Geometry: final body of the model. Coordinates: model frame, mm. Face numbers are marked on the shaded views. A direction names the side the tool comes from. Round coordinates to 2 decimals unless told otherwise and drop trailing zeros. Loops run counter-clockwise (first coordinate to the right, second up) from the corner with the lowest first, then second, coordinate; pieces in that order, holes last. Notation, with made-up numbers: M 30,13.25 L 55,13.25 A14 cw 55,26.25 Z; hole C 8,-7.75 d1. An arc over 180 degrees is marked long. Return JSON: item names as keys, results as strings.
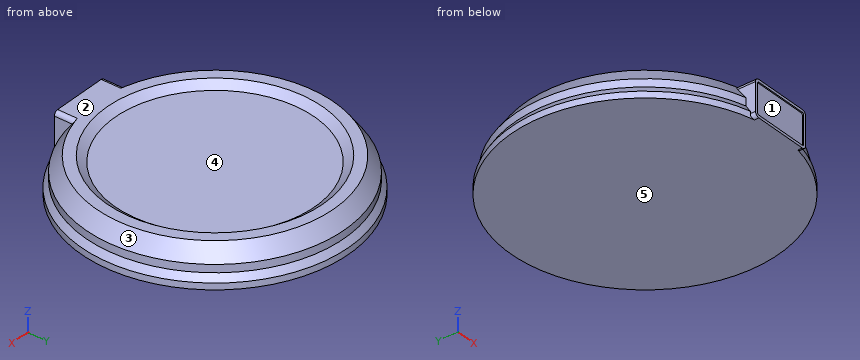
from build123d import *

# Parameters (mm, degrees)
F3_W     = 38
F3_H     = 19.3329955554
F4_DEPTH = 12.3
F5_DEPTH = 3.5
F6_DEPTH = 2.7745664948
F7_R     = 2.5
F9_DEPTH = 0.7


with BuildPart() as f1:
    # F0 (on Front) → F1 (revolve)
    with BuildSketch(Plane.XZ):
        Polygon((0, 18.3759443462), (0, 0), (81.9731503725, 0), (81.9731503725, 3.9145960473), (79.3440267444, 8.0617284402), (79.3440267444, 12.8429912047), (72.8131681681, 22.1075620502), (66.1219879985, 22.1075620502), (61.1036121845, 18.3759443462), align=None)
    revolve(axis=Axis((0, 0, 9.1879721731), (0, 0, 1)))

    # F3 (on offset) → F4 (join)
    with BuildSketch(Plane.XZ.offset(79.48)):
        with Locations((0, 12.4410642725)):
            Rectangle(F3_W, F3_H)
    extrude(amount=-F4_DEPTH)

    # F3 (on offset) → F5 (join)
    with BuildSketch(Plane.XZ.offset(79.48)):
        with Locations((0, 12.4410642725)):
            Rectangle(F3_W, F3_H)
    extrude(amount=F5_DEPTH)

    # F6 (add, through all): a face of the model
    f6_faces = [f1.faces().sort_by_distance(p)[0] for p in [
        (0, -81.9802862149, 2.7745664948),
    ]]
    extrude(f6_faces, amount=F6_DEPTH)

    # F7
    f7_edges = [f1.edges().sort_by_distance(p)[0] for p in [
        (-19, -76.635261, 22.107562),
        (19, -76.635261, 22.107562),
        (19, -81.360407, 0),
        (-19, -81.360407, 0),
    ]]
    fillet(f7_edges, radius=F7_R)

    # F8 (on face) → F9 (cut)
    with BuildSketch(Plane.XZ.offset(82.98)):
        with BuildLine():
            Line((16.5, 20.5075629056), (-16.5, 20.5075629056))
            ThreePointArc((-16.5, 20.5075629056), (-17.1363967079, 20.2439587581), (-17.4000008553, 19.6075620502))
            Line((-17.4000008553, 19.6075620502), (-17.4000008553, 2.5))
            ThreePointArc((-17.4000008553, 2.5), (-17.1363967079, 1.8636032921), (-16.5, 1.5999991447))
            Line((-16.5, 1.5999991447), (16.5, 1.5999991447))
            ThreePointArc((16.5, 1.5999991447), (17.1363967079, 1.8636032921), (17.4000008553, 2.5))
            Line((17.4000008553, 2.5), (17.4000008553, 19.6075620502))
            ThreePointArc((17.4000008553, 19.6075620502), (17.1363967079, 20.2439587581), (16.5, 20.5075629056))
        make_face()
    extrude(amount=-F9_DEPTH, mode=Mode.SUBTRACT)


solid = f1.part
Q1. Section query A-A (x = 0). Output: boundary loops of the cut face in (y, z), plus the area to 3 significant figures.
Determined:
{"outline": "M -82.98,0 L 81.97,0 L 81.97,3.91 L 79.34,8.06 L 79.34,12.84 L 72.81,22.11 L 66.12,22.11 L 61.1,18.38 L -61.1,18.38 L -66.12,22.11 L -82.98,22.11 L -82.98,20.51 L -82.28,20.51 L -82.28,1.6 L -82.98,1.6 Z", "area": "3,090 mm^2"}
Q2. Pin query (flat end, axial travel): pin 1 (10 mm diameter, centred on y = 15.5, z = 14, fed in from -X); pin 2 (10 mm diameter, centred on y = 41, z = 12, fed in from -X); pin 3 (10 mm diameter, centred on x = -47.5, z = 11, fed in from -Y). Return the tip coordinate at first contact, or that it passes through.
Determined:
{"pin 1": "stops at x = -78.63", "pin 2": "stops at x = -70.71", "pin 3": "stops at y = -67"}
Q3. Reachability of the marked faces 4 and 5 from +Z, -Z, +X, -X, +Y, -Y: full face, straight path, thin tool, end or side. Return the list, or none.
Determined:
{"face 4": "+Z", "face 5": "-Z, +X, -X, +Y, -Y"}
Q4. Pull-direction query (X, two-part tool) for the marked faces 1, 2 and 3; classes: pulls with the +X half, pulls with the -X half, needs draft (parallel to the pull), parting line crosses it, or undercut.
Determined:
{"face 1": "undercut", "face 2": "needs draft", "face 3": "parting line crosses it"}
Q5. Section query C-C (z = 15.25). Output: boundary loops of the cut face in (x, y), plus the area to 3 significant figures.
Determined:
{"outline": "M -19,-82.98 L -17.4,-82.98 L -17.4,-82.28 L 17.4,-82.28 L 17.4,-82.98 L 19,-82.98 L 19,-75.29 A77.65 ccw long -19,-75.29 Z", "area": "19,100 mm^2"}
Q6. Section query B-B (y = 0). Output: boundary loops of the cut face in (x, z).
Determined:
{"outline": "M -81.97,0 L 81.97,0 L 81.97,3.91 L 79.34,8.06 L 79.34,12.84 L 72.81,22.11 L 66.12,22.11 L 61.1,18.38 L -61.1,18.38 L -66.12,22.11 L -72.81,22.11 L -79.34,12.84 L -79.34,8.06 L -81.97,3.91 Z"}
Q7. Material intervals for L1, parallel to Z at x = 47.5, y = 3; L2, parallel to Y at x = 49, z = 19.25; L3, parallel to Y at x = 24.5, z = 21, sorted ascending.
Determined:
{"L1": "z = 0 to 18.38", "L2": "y = -56.55 to -38.44, 38.44 to 56.55", "L3": "y = -69.4 to -59.81, 59.81 to 69.4"}
